Can you work these out from the model? Positions are in its coordinate system, mm. A direction names the side the tool comes from. Coordinates: 2 decimals unless noted, no trailing zeros. Order: outer loops, then holes, each group sorted by start corner. A loop starts at its lowest first (then second) coordinate and runs counter-clockwise, first axis right, second up. Notation, with made-up numbers: (24.25, -36) - (67.25, -36) arc R19 cw to (67.25, -28) - close; hole circle Ø3 at (-36, 63). An arc over 180 degrees is marked (long way). Return JSON: item names as keys, results as strings. Group by question number.
1) Imagine slicing it at C-C (z = -5.75). Write out the boundary of the cut face in (x, y), and give its area (3 significant figures).
2) If I drill on line 1 along X through (y, z) = (-26.6, -10); line 2 along Z through (x, y) = (-6, -26.55); line 3 along Y through (x, z) = (-14.5, -7.5), over which ranges is the centre line in solid material (lowest first)?
3) Imagine slicing it at B-B (x = 6). Write out the boundary of the cut face in (y, z).
4) If we mould it in two halves opening along Z, with no side actions, what happens to faces 1 (the face through (0, 0, 4)), 2 (the face through (0, 2, 0)), 3 (the face through (-5.63, -26.74, -8.34)), 4 (the face through (0, -28, -8))? For each: pulls with the +Z half, pulls with the -Z half, needs draft (parallel to the pull), parting line crosses it, or undercut.
5) Which directions (+Z, -Z, +X, -X, +Y, -Y) give clear straight access to the entire face, cutting with the end or side of a thin tool? Please do faces 5 (the face through (0, -24, -10)), 6 (the face through (0, 28, 2)).
6) For pin 1 Ø12 at (x, y) = (-5, -14) entering from -Z; pin 2 Ø6 at (x, z) = (-10, -5.5) entering from +Y, each with a flat end and sliding along its axis, tell me the tip position at first contact or that it passes through.
7) Imagine slicing it at A-A (z = -10). Write out the boundary of the cut face in (x, y).
8) Imagine slicing it at D-D (x = 11). Write out the boundary of the cut face in (y, z), and give its area (3 significant figures).
```python
from build123d import *

# Parameters (mm, degrees)
SKETCH1_W                                           = 36
SKETCH1_H                                           = 56
BOSS_EXTRUDE1_DEPTH                                 = 4
SKETCH2_W                                           = 36
SKETCH2_H                                           = 4
BOSS_EXTRUDE2_DEPTH                                 = 20
CSK_FOR_M3_COUNTERSUNK_FLAT_HEAD_SCREW1_D           = 3.4
CSK_FOR_M3_COUNTERSUNK_FLAT_HEAD_SCREW1_CSINK_D     = 6.3
CSK_FOR_M3_COUNTERSUNK_FLAT_HEAD_SCREW1_CSINK_ANGLE = 90


with BuildPart() as part:
    # Sketch1 → Boss-Extrude1 (new body)
    with BuildSketch(Plane.XY):
        Rectangle(SKETCH1_W, SKETCH1_H)
    extrude(amount=BOSS_EXTRUDE1_DEPTH)

    # Sketch2 → Boss-Extrude2 (add)
    with BuildSketch(Plane(origin=(0, 0, 0), x_dir=(-1, 0, 0), z_dir=(0, 0, -1))):
        with Locations((0, -26)):
            Rectangle(SKETCH2_W, SKETCH2_H)
    extrude(amount=BOSS_EXTRUDE2_DEPTH)

    # CSK for M3 Countersunk Flat Head Screw1 (through all)
    with Locations(Plane(origin=(0, -24, 0), x_dir=(1, 0, 0), z_dir=(0, 1, 0))):
        with Locations((6, 10), (-6, 10)):
            CounterSinkHole(CSK_FOR_M3_COUNTERSUNK_FLAT_HEAD_SCREW1_D / 2, CSK_FOR_M3_COUNTERSUNK_FLAT_HEAD_SCREW1_CSINK_D / 2, counter_sink_angle=CSK_FOR_M3_COUNTERSUNK_FLAT_HEAD_SCREW1_CSINK_ANGLE)


solid = part.part
```
Calculated:
{
 "1": {"outline": "(-18, -28) - (18, -28) - (18, -24) - (-18, -24) - close", "area": "144 mm2"},
 "2": {"line 1": "-18 to -7.7, -4.3 to 4.3, 7.7 to 18", "line 2": "-20 to -11.7, -8.3 to 4", "line 3": "-28 to -24"},
 "3": {"outline": "(-28, -20) - (-24, -20) - (-24, -13.15) - (-25.45, -11.7) - (-28, -11.7) - close; (-28, -8.3) - (-25.45, -8.3) - (-24, -6.85) - (-24, 0) - (28, 0) - (28, 4) - (-28, 4) - close"},
 "4": {"face 1": "pulls with the +Z half", "face 2": "pulls with the -Z half", "face 3": "undercut", "face 4": "needs draft"},
 "5": {"face 5": "-Z, +X, -X, +Y", "face 6": "+Z, -Z, +X, -X, +Y"},
 "6": {"pin 1": "z = 0", "pin 2": "y = -24"},
 "7": {"outline": "(-18, -28) - (-7.7, -28) - (-7.7, -25.45) - (-9.15, -24) - (-18, -24) - close; (-4.3, -28) - (4.3, -28) - (4.3, -25.45) - (2.85, -24) - (-2.85, -24) - (-4.3, -25.45) - close; (7.7, -28) - (18, -28) - (18, -24) - (9.15, -24) - (7.7, -25.45) - close"},
 "8": {"outline": "(-28, -20) - (-24, -20) - (-24, 0) - (28, 0) - (28, 4) - (-28, 4) - close", "area": "304 mm2"}
}
